from build123d import *

# Parameters (mm, degrees)
F0_R        = 61.35
F0_R_2      = 1.25
F0_R_3      = 5.5
F1_DEPTH    = 2
F2_R        = 61.35
F2_R_2      = 60.75
F3_DEPTH    = 37
F2_R_3      = 59.75
F4_DEPTH    = 26
F5_DEPTH    = 25
F6_S5_R     = 59.75
F6_T6_DEPTH = 87
F7_SIZE     = 5
F8_DEPTH    = 1


# Not quite as in the source:
# - a fillet or chamfer that OpenCascade refuses, or shapes differently, is made with other operations: its cross-section is extruded or revolved along the edge and cut away or added


with BuildPart() as f1:
    # F0 (on Top) → F1 (new body)
    with BuildSketch(Plane.XY):
        Circle(F0_R)
        with Locations((17, -29.4448637287)):
            Circle(F0_R_2, mode=Mode.SUBTRACT)
        with Locations((-34, 0)):
            Circle(F0_R_2, mode=Mode.SUBTRACT)
        Circle(F0_R_3, mode=Mode.SUBTRACT)
        with Locations((17, 29.4448637287)):
            Circle(F0_R_2, mode=Mode.SUBTRACT)
    extrude(amount=F1_DEPTH)

    # F2 (on face) → F3 (join)
    with BuildSketch(Plane.XY.offset(2)):
        Circle(F2_R)
        Circle(F2_R_2, mode=Mode.SUBTRACT)
    extrude(amount=F3_DEPTH)

    # F2 (on face) → F4 (join)
    with BuildSketch(Plane.XY.offset(2)):
        Circle(F2_R_2)
        Circle(F2_R_3, mode=Mode.SUBTRACT)
    extrude(amount=F4_DEPTH)

    # F2 (on face) → F5 (cut)
    with BuildSketch(Plane.XY.offset(2)):
        Circle(F2_R_2)
        Circle(F2_R_3, mode=Mode.SUBTRACT)
    extrude(amount=F5_DEPTH, mode=Mode.SUBTRACT)

    # F6: chamfer of 2 on 1 edges, made by hand


with BuildPart() as f6_tool2:
    # F6_s3 → F6_t4 (revolve)
    with BuildSketch(Plane.XZ):
        Polygon((60.75, 25), (58.75, 27), (60.75, 27), align=None)
    revolve(axis=Axis((0, 0, 27), (0, 0, 1)))

    # F6_s5 → F6_t6 (cut, symmetric)
    with BuildSketch(Plane.XY.offset(26)):
        Circle(F6_S5_R)
    extrude(amount=F6_T6_DEPTH, both=True, mode=Mode.SUBTRACT)


with BuildPart() as f1_1:
    add(f1.part)

    # F6_t1: union F6_tool2
    add(f6_tool2.part)

    # F7
    f7_edges = [f1_1.edges().sort_by_distance(p)[0] for p in [
        (-60.75, 0, 2),
    ]]
    chamfer(f7_edges, length=F7_SIZE)

    # F8 (cut): a face of the model
    f8_faces = [f1_1.faces().sort_by_distance(p)[0] for p in [
        (-59.614759959, 0, 0),
    ]]
    extrude(f8_faces, amount=-F8_DEPTH, mode=Mode.SUBTRACT)


solid = f1_1.part
Build history of the part. All positions in model axes, mm. A direction names the side the tool comes from. Round coordinates to 2 decimals unless told otherwise and drop trailing zeros. Loops run counter-clockwise (first coordinate to the right, second up) from the corner with the lowest first, then second, coordinate; pieces in that order, holes last. Notation, with made-up numbers: (-30.75, 45.25) -> (18.25, 45.25) arc R17 cw to (18.25, 71.25) -> close; hole circle Ø10 at (-9.75, 23.25). An arc over 180 degrees is marked (long way). One line per item, written item: value. Start each with the question number.
Q1. Drop flat-ended pins along their axis: pin 1 Ø12.5 at (x, y) = (0, 0) entering from -Z; pin 2 Ø2 at (x, y) = (-46, 11) entering from +Z; pin 3 Ø1 at (x, z) = (33.5, 26.5) entering from -Y; pin 4 Ø8 at (x, z) = (36.5, 18) entering from -Y. Give the stop position or say it passes through.
Q2. Cut at B-B on z = 3.5. List the corners of the cut face in (x, y).
Q3. 3-axis set-ups, long thin cutter, end or side, ignore diameter. For faces 1 (the face through (53.407, 16.819, 2.243)), 2 (the face through (55.194, -22.885, 27.014)), 3 (the face through (-1.19, -5.37, 1.49)): which of +Z, -Z, +X, -X, +Y, -Y reach the whole face in a straight line?
Q4. Cut at A-A on x = 0. List the corners of the cut face in (y, z).
Q5. Two-plate mould, pull along Y, no slides. Class faces 4 (the face through (-61.29, 2.7, 19.73)), 5 (the face through (57.945, 18.248, 15.874)), 6 (the face through (-13.9, 59.4, 39)): released by +Y, released by -Y, zero draft, split by the parting line, or undercut.
Q6. Probe line 1 along Y through (x, z) = (17, 1.3); line 2 along Y through (x, z) = (0, 35); line 3 along Z through (x, y) = (2.5, 8). List the from-to ranges inside material, lowest first.
Computed:
1. pin 1: z = 1
1. pin 2: z = 2
1. pin 3: y = -51.72
1. pin 4: y = -52.03
2. outline: circle Ø122.7 at (0, 0); hole circle Ø114.5 at (0, 0)
3. face 1: none
3. face 2: +Z
3. face 3: +Z, -Z
4. outline: (-61.35, 1) -> (-5.5, 1) -> (-5.5, 2) -> (-55.75, 2) -> (-60.75, 7) -> (-60.75, 25) -> (-59.75, 26) -> (-59.75, 28) -> (-60.75, 28) -> (-60.75, 39) -> (-61.35, 39) -> close; (5.5, 1) -> (61.35, 1) -> (61.35, 39) -> (60.75, 39) -> (60.75, 28) -> (59.75, 28) -> (59.75, 26) -> (60.75, 25) -> (60.75, 7) -> (55.75, 2) -> (5.5, 2) -> close
5. face 4: split by the parting line
5. face 5: undercut
5. face 6: zero draft
6. line 1: -58.95 to -30.69, -28.19 to 28.19, 30.69 to 58.95
6. line 2: -61.35 to -60.75, 60.75 to 61.35
6. line 3: 1 to 2
